Verification items for the finished model (mm, model axes). A direction names the side the tool comes from. Give positions to 0.01 mm unless a question says otherwise; leave off trailing zeros. Write each loop counter-clockwise with the first axis right and the second up, starting at its lowest first coordinate (ties: lowest second). Pieces come first, ordered by that corner, then holes. Notation, with made-up numbers: (28.25, -37) - (64.25, -37) arc R15 cw to (64.25, -27) - close; hole circle Ø4 at (24.25, -23.5). An arc over 180 degrees is marked (long way). Put each result on its own line as item: value.
Autodesk Inventor part; units mm, degrees
ref_plane "YZ Plane" through (0, 0, 0) normal (1, 0, 0) x (0, 1, 0)
ref_plane "XZ Plane" through (0, 0, 0) normal (0, 1, 0) x (-1, 0, 0)
ref_plane "XY Plane" through (0, 0, 0) normal (0, 0, 1) x (1, 0, 0)
sketch "Sketch1" plane through (0, 0, 0) normal (0, 0, 1) x (1, 0, 0)
  line L0 (0, 0) -> (50.8, 0) construction
  line L1 (50.8, 0) -> (50.8, 127) construction
  line L2 (50.8, 127) -> (0, 127) construction
  line L3 (0, 127) -> (0, 0) construction
  line L4 (0, 63.5) -> (50.8, 63.5) construction
  line L5 (25.4, 127) -> (25.4, 0) construction
  line L6 (6.7469, 46) -> (44.0531, 46) construction
  line L7 (44.0531, 46) -> (44.0531, 81) construction
  line L8 (44.0531, 81) -> (6.7469, 81) construction
  line L9 (6.7469, 81) -> (6.7469, 46) construction
  line L10 (41.6177, 127) -> (41.6177, 0) construction
  line L11 (26.6177, 127) -> (26.6177, 0) construction
  line L12 (45.2437, 28.575) -> (45.2437, 98.425)
  line L13 (45.2437, 98.425) -> (22.9917, 98.425)
  line L14 (22.9917, 98.425) -> (22.9917, 28.575)
  line L15 (22.9917, 28.575) -> (45.2437, 28.575)
  line L16 (42.0688, 28.575) -> (42.0688, 98.425)
  line L17 (26.1667, 28.575) -> (26.1667, 98.425)
  line L18 (24.5927, 22.225) -> (43.6427, 22.225)
  line L19 (43.6427, 22.225) -> (43.6427, 15.875)
  line L20 (43.6427, 15.875) -> (24.5927, 15.875)
  line L21 (24.5927, 15.875) -> (24.5927, 22.225)
  line L22 (34.1177, 0) -> (34.1177, 127) construction
  line L23 (43.6427, 111.125) -> (24.5927, 111.125)
  line L24 (24.5927, 111.125) -> (24.5927, 104.775)
  line L25 (24.5927, 104.775) -> (43.6427, 104.775)
  line L26 (43.6427, 104.775) -> (43.6427, 111.125)
  line L27 (19.8302, 12.7) -> (48.4052, 12.7)
  line L28 (48.4052, 12.7) -> (48.4052, 114.3)
  line L29 (48.4052, 114.3) -> (19.8302, 114.3)
  line L30 (19.8302, 114.3) -> (19.8302, 12.7)
  dimension "d0" = 50.8
  dimension "d1" = 127
  dimension "d2" = 35
  dimension "d3" = 37.3062
  dimension "d4" = 15
  dimension "d5" = 2.4354
  dimension "d6" = 5.5563
  dimension "d7" = 3.175
  dimension "d8" = 0.451
  dimension "d9" = 0.451
  dimension "d10" = 3.175
  dimension "d11" = 69.85
  dimension "d12" = 19.05
  dimension "d13" = 6.35
  dimension "d14" = 6.35
  dimension "d15" = 6.35
  dimension "d16" = 19.05
  dimension "d17" = 6.35
  dimension "d18" = 3.175
  dimension "d21" = 3.175
  dimension "d30" = 28.575
  dimension "d32" = 3.1615
  dimension "d33" = 3.1615
extrude "Main Cover Profile" add sketch "Sketch1" along normal blind 4.7625 contours L15 L16 L13 L12 | L15 L17 L13 L16 | L15 L14 L13 L17 | L18 L19 L20 L21 | L26 L25 L24 L23 | L30 L29 L28 L27
extrude "Magnet Pockets" cut sketch "Sketch1" along normal blind 2.3813 contours L18 L19 L20 L21 | L26 L25 L24 L23
extrude "Belt Aligning Tabs" add sketch "Sketch1" against normal blind 12.7 contours L15 L16 L13 L12 | L15 L14 L13 L17
fillet "Fillet1" radius 3.175 8 edges at (43.6427, 22.225, 1.1906) (43.6427, 15.875, 1.1906) (24.5927, 15.875, 1.1906) (24.5927, 22.225, 1.1906) (43.6427, 104.775, 1.1906) (43.6427, 111.125, 1.1906) (24.5927, 104.775, 1.1906) (24.5927, 111.125, 1.1906)
equation "\"d5\" = -0.666667 * d4 + 0.333333 * d3"
equation "\"d9\" = d8"
equation "\"d10\" = d7"
equation "\"d12\" = d16"
equation "\"d13\" = d15"
properties part number "Belt Aligner MagLock" material "Polyethylene, High Density"
Q1. Section check A-A, the plane z = -11. Record the cut outline in (x, y) (3 decimals).
Answers follow:
outline: (22.992, 28.575) - (26.167, 28.575) - (26.167, 98.425) - (22.992, 98.425) - close; (42.069, 28.575) - (45.244, 28.575) - (45.244, 98.425) - (42.069, 98.425) - close
Q2. Release check for a two-part mould opening along X. For faces 5 (the face through (34, 111.125, 1)), 6 (the face through (34, 64, 4.762)), 7 (the face through (45.244, 63, -6)) record: released by +X, released by -X, zero draft, split by the parting line, or undercut.
Answers follow:
face 5: undercut
face 6: zero draft
face 7: released by +X
Q3. Section check C-C, the plane y = 64.5. Record the cut outline in (x, z).
Answers follow:
outline: (19.83, 0) - (22.99, 0) - (22.99, -12.7) - (26.17, -12.7) - (26.17, 0) - (42.07, 0) - (42.07, -12.7) - (45.24, -12.7) - (45.24, 0) - (48.41, 0) - (48.41, 4.76) - (19.83, 4.76) - close
Q4. Go/stop test with flat-tipped pins: pin 1 Ø1.9 at (x, y) = (32.5, 106.5) entering from -Z; pin 2 Ø2.5 at (x, z) = (44, -8.5) entering from +Y (3 decimals); pin 3 Ø1.5 at (y, z) = (84.5, -10) entering from +X. Record where each tip stops, or that it passes through.
Answers follow:
pin 1: stops at z = 2.38
pin 2: stops at y = 98.425
pin 3: stops at x = 45.24
Q5. Scan lines: line 1 along Y through (x, z) = (30, 1.75) (3 decimals); line 2 along X through (y, z) = (65.5, -6.75); line 3 along Z through (x, y) = (40.25, 38). Record each from-to range of solid material in increasing order.
Answers follow:
line 1: y = 12.7 to 15.875, 22.225 to 104.775, 111.125 to 114.3
line 2: x = 22.99 to 26.17, 42.07 to 45.24
line 3: z = 0 to 4.76
Q6. Set-up check for faces 1 (the face through (25.5, 105.73, 1.21)), 2 (the face through (44, 98.425, -6)), 3 (the face through (22.992, 64, -6)), 4 (the face through (42.069, 63, -6)): record each of +Z, -Z, +X, -X, +Y, -Y from which the full face is reachable in a straight line by a thin tool's end or side.
Answers follow:
face 1: -Z
face 2: -Z, +X, -X, +Y
face 3: -Z, -X, +Y, -Y
face 4: -Z, +Y, -Y
Q7. Section check B-B, the plane x = 34. Record the cut outline in (y, z) (1 decimal).
Answers follow:
outline: (12.7, 0) - (15.9, 0) - (15.9, 2.4) - (22.2, 2.4) - (22.2, 0) - (104.8, 0) - (104.8, 2.4) - (111.1, 2.4) - (111.1, 0) - (114.3, 0) - (114.3, 4.8) - (12.7, 4.8) - close
